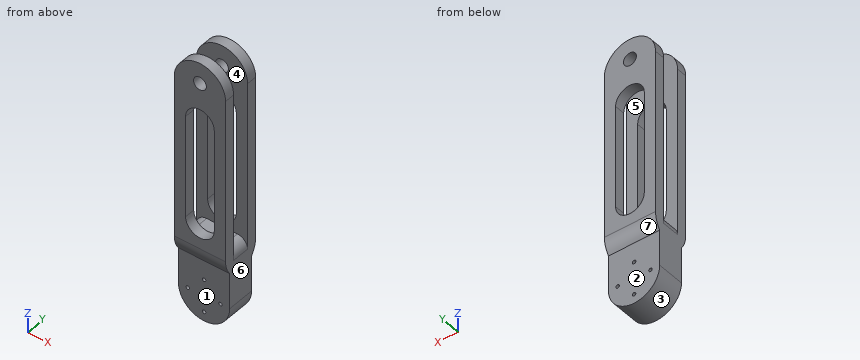
```python
from build123d import *

# Parameters (mm, degrees)
BOSS_EXTRU_1_DEPTH      = 12.5
CONG_1_R                = 12.5
ESQUISSE2_R             = 0.85
ENL_V_MAT_EXTRU_1_DEPTH = 122.715469949
ESQUISSE3_R             = 3.15
ENL_V_MAT_EXTRU_2_DEPTH = 123.082236628
ENL_V_MAT_EXTRU_3_DEPTH = 123.082236628
CONG_2_R                = 5


with BuildPart() as part:
    # Esquisse1 → Boss.-Extru.1 (new, symmetric)
    with BuildSketch(Plane(origin=(0, 0, 0), x_dir=(0, 0, -1), z_dir=(1, 0, 0))):
        Polygon((90, 9.325), (-10, 9.325), (-10, 4.325), (80, 4.325), (80, -4.325), (-10, -4.325), (-10, -9.325), (90, -9.325), (90, -6.75), (120, -6.75), (120, 6.75), (90, 6.75), align=None)
    extrude(amount=BOSS_EXTRU_1_DEPTH, both=True)

    # Congé1
    # the kernel refuses this fillet: 12.5 mm, written as the material it takes off along each edge
    with BuildSketch(Plane(origin=(-31.497429925, -9.325, -90), x_dir=(0, 1, 0), z_dir=(1, 0, 0))) as cong_1_piece_1:
        with BuildLine():
            CenterArc((12.5, 7.59897197), CONG_1_R, 180, 37.439095089)
            Line((0, 7.59897197), (-0.25, 7.59897197))
            Line((-0.25, 7.59897197), (-0.25, 0))
            Line((-0.25, 0), (0, -0.25))
            ThreePointArc((0, -0.25), (1.2875, -0.25), (2.3765, -0.151979439))
            Line((2.3765, -0.151979439), (2.575, 0))
        make_face()
    extrude(amount=62.99485985, mode=Mode.SUBTRACT)
    with BuildSketch(Plane(origin=(31.497429925, 9.325, -90), x_dir=(0, 0, 1), z_dir=(-1, 0, 0))) as cong_1_piece_2:
        with BuildLine():
            CenterArc((7.59897197, -12.5), CONG_1_R, 90, 37.439095089)
            Line((0, -2.575), (-0.151979439, -2.3765))
            ThreePointArc((-0.151979439, -2.3765), (-0.25, -1.2875), (-0.25, 0))
            Line((-0.25, 0), (0, 0.25))
            Line((0, 0.25), (7.59897197, 0.25))
            Line((7.59897197, 0.25), (7.59897197, 0))
        make_face()
    extrude(amount=62.99485985, mode=Mode.SUBTRACT)
    with BuildSketch(Plane(origin=(-12.5, 26.925, 10), x_dir=(1, 0, 0), z_dir=(0, -1, 0)), Plane(origin=(-12.5, 40.575, 10), x_dir=(1, 0, 0), z_dir=(0, -1, 0)), Plane(origin=(12.5, 40.575, 10), x_dir=(0, 0, -1), z_dir=(0, -1, 0))) as cong_1_piece_3:
        with BuildLine():
            CenterArc((CONG_1_R, -CONG_1_R), CONG_1_R, 90, 90)
            Line((0, -CONG_1_R), (-CONG_1_R * 0.02, -CONG_1_R))
            Line((-CONG_1_R * 0.02, -CONG_1_R), (-CONG_1_R * 0.02, CONG_1_R * 0.02))
            Line((-CONG_1_R * 0.02, CONG_1_R * 0.02), (CONG_1_R, CONG_1_R * 0.02))
            Line((CONG_1_R, CONG_1_R * 0.02), (CONG_1_R, 0))
        make_face()
    extrude(amount=67.5, mode=Mode.SUBTRACT)
    with BuildSketch(Plane(origin=(12.5, 26.925, 10), x_dir=(-1, 0, 0), z_dir=(0, -1, 0))) as cong_1_piece_4:
        with BuildLine():
            CenterArc((CONG_1_R, CONG_1_R), CONG_1_R, 180, 90)
            Line((0, CONG_1_R), (-CONG_1_R * 0.02, CONG_1_R))
            Line((-CONG_1_R * 0.02, CONG_1_R), (-CONG_1_R * 0.02, -CONG_1_R * 0.02))
            Line((-CONG_1_R * 0.02, -CONG_1_R * 0.02), (CONG_1_R, -CONG_1_R * 0.02))
            Line((CONG_1_R, -CONG_1_R * 0.02), (CONG_1_R, 0))
        make_face()
    extrude(amount=67.5, mode=Mode.SUBTRACT)
    with BuildSketch(Plane(origin=(-12.5, -38, -120), x_dir=(1, 0, 0), z_dir=(0, 1, 0))) as cong_1_piece_5:
        with BuildLine():
            CenterArc((CONG_1_R, -CONG_1_R), CONG_1_R, 90, 90)
            Line((0, -CONG_1_R), (-CONG_1_R * 0.02, -CONG_1_R))
            Line((-CONG_1_R * 0.02, -CONG_1_R), (-CONG_1_R * 0.02, CONG_1_R * 0.02))
            Line((-CONG_1_R * 0.02, CONG_1_R * 0.02), (CONG_1_R, CONG_1_R * 0.02))
            Line((CONG_1_R, CONG_1_R * 0.02), (CONG_1_R, 0))
        make_face()
    extrude(amount=76, mode=Mode.SUBTRACT)
    with BuildSketch(Plane(origin=(12.5, -38, -120), x_dir=(-1, 0, 0), z_dir=(0, 1, 0))) as cong_1_piece_6:
        with BuildLine():
            CenterArc((CONG_1_R, CONG_1_R), CONG_1_R, 180, 90)
            Line((0, CONG_1_R), (-CONG_1_R * 0.02, CONG_1_R))
            Line((-CONG_1_R * 0.02, CONG_1_R), (-CONG_1_R * 0.02, -CONG_1_R * 0.02))
            Line((-CONG_1_R * 0.02, -CONG_1_R * 0.02), (CONG_1_R, -CONG_1_R * 0.02))
            Line((CONG_1_R, -CONG_1_R * 0.02), (CONG_1_R, 0))
        make_face()
    extrude(amount=76, mode=Mode.SUBTRACT)

    # Esquisse2 → Enlèv. mat.-Extru.1 (cut, through all)
    with BuildSketch(Plane(origin=(0, 6.75, 0), x_dir=(1, 0, 0), z_dir=(0, 1, 0))):
        with Locations(Location((8, 107.5, 0), (0, 0, 270))):
            Circle(ESQUISSE2_R)
        with Locations(Location((0, 115.5, 0), (0, 0, 270))):
            Circle(ESQUISSE2_R)
        with Locations(Location((-8, 107.5, 0), (0, 0, 270))):
            Circle(ESQUISSE2_R)
        with Locations(Location((0, 99.5, 0), (0, 0, 270))):
            Circle(ESQUISSE2_R)
    extrude(amount=-ENL_V_MAT_EXTRU_1_DEPTH, mode=Mode.SUBTRACT)

    # Esquisse3 → Enlèv. mat.-Extru.2 (cut, through all)
    with BuildSketch(Plane(origin=(0, 9.325, 0), x_dir=(1, 0, 0), z_dir=(0, 1, 0))):
        with Locations(Location((0, 0, 0), (0, 0, 270))):
            Circle(ESQUISSE3_R)
    extrude(amount=-ENL_V_MAT_EXTRU_2_DEPTH, mode=Mode.SUBTRACT)

    # Esquisse4 → Enlèv. mat.-Extru.3 (cut, through all)
    with BuildSketch(Plane(origin=(0, 9.325, 0), x_dir=(1, 0, 0), z_dir=(0, 1, 0))):
        with BuildLine():
            Line((-7, 70), (-7, 20))
            ThreePointArc((-7, 20), (0, 13), (7, 20))
            Line((7, 20), (7, 70))
            ThreePointArc((7, 70), (0, 77), (-7, 70))
        make_face()
    extrude(amount=-ENL_V_MAT_EXTRU_3_DEPTH, mode=Mode.SUBTRACT)

    # Congé2
    cong_2_edges = [part.edges().sort_by_distance(p)[0] for p in [
        (12.5, 0, -80),
        (-12.5, 0, -80),
    ]]
    fillet(cong_2_edges, radius=CONG_2_R)


solid = part.part
```
The model under review builds one solid part; all positions refer to its coordinate system, in mm. Face numbers are marked on the shaded views. A direction names the side the tool comes from. Give positions to 0.01 mm unless a question says otherwise; leave off trailing zeros. Write each loop counter-clockwise with the first axis right and the second up, starting at its lowest first coordinate (ties: lowest second). Pieces come first, ordered by that corner, then holes. Notation, with made-up numbers: (66.5, -17) - (80.5, -17) arc R19 ccw to (80.5, 15) - close; hole circle Ø8 at (31.5, 31.5). An arc over 180 degrees is marked (long way). Answer in a Markdown table with one row per item. Add a question column.
1. Wall thickness on line 1 along X through (y, z) = (3.5, -107.5); line 2 along Y through (x, z) = (4.5, -9) (3 decimals); line 3 along X through (y, z) = (-7.5, -55): over which ranges is each line inside the solid? List them lowest first. Write a range as [from, to].
2. Draft analysis for pull direction Y (two halves, no side actions). For the marked faces 4, 5, 6 and 7, state which applies: +Y half, -Y half, draft (parallel to the pull), parting line (faces both ways), or undercut.
3. Tool access review of the marked faces 1, 2 and 3: name each direction out of +Z, -Z, +X, -X, +Y, -Y from which nothing blocks a thin tool from reaching the whole face with its end or side.
4. Insertion check: P1, Ø4, axis at x = 8, z = -93, coming from the +Y side; P2, Ø4.5, axis at x = 3.5, y = -1, coming from the +Z side; P3, Ø2, axis at x = -8, z = -107.5, coming from the -Y side. Each pin has a flat end and moves straight along its axis. Give the tip position at first contact, or say it passes through.
5. We need section D-D on z = 1. Write out the cut boundary in (x, y) (3 decimals), then the cut area to 3 significant figures.
6. We need section C-C on x = 4.5. Write out the cut boundary in (y, z) (3 decimals), then the cut area to 3 significant figures.
7. We need section A-A on z = -26.5. Write out the cut boundary in (x, y) (3 decimals).
8. We need section B-B on y = 5.5. Write out the cut boundary in (x, z).
Ans:
| question | item | result |
|---|---|---|
| 1 | line 1 | x = [-12.5, -8.85], [-7.15, 7.15], [8.85, 12.5] |
| 1 | line 2 | y = [-9.325, -4.325], [4.325, 9.325] |
| 1 | line 3 | x = [-12.5, -7], [7, 12.5] |
| 2 | face 4 | undercut |
| 2 | face 5 | undercut |
| 2 | face 6 | draft |
| 2 | face 7 | +Y half |
| 3 | face 1 | -Z, +X, -X, -Y |
| 3 | face 2 | -Z, +X, -X, +Y |
| 3 | face 3 | -Z, +Y, -Y |
| 4 | P1 | stops at y = 6.75 |
| 4 | P2 | stops at z = -80 |
| 4 | P3 | stops at y = -6.75 |
| 5 | outline | (-12, -9.325) - (-2.987, -9.325) - (-2.987, -4.325) - (-12, -4.325) - close; (-12, 4.325) - (-2.987, 4.325) - (-2.987, 9.325) - (-12, 9.325) - close; (2.987, -9.325) - (12, -9.325) - (12, -4.325) - (2.987, -4.325) - close; (2.987, 4.325) - (12, 4.325) - (12, 9.325) - (2.987, 9.325) - close |
| 5 | area | 180 mm^2 |
| 6 | outline | (-9.325, -82.401) arc R12.5 ccw to (-6.75, -90) - (-6.75, -119.162) - (6.75, -119.162) - (6.75, -90) arc R12.5 ccw to (9.325, -82.401) - (9.325, -75.362) - (4.325, -75.362) - (4.325, -80) - (-4.325, -80) - (-4.325, -75.362) - (-9.325, -75.362) - close; (-9.325, -14.638) - (-4.325, -14.638) - (-4.325, 9.162) - (-9.325, 9.162) - close; (4.325, -14.638) - (9.325, -14.638) - (9.325, 9.162) - (4.325, 9.162) - close |
| 6 | area | 852 mm^2 |
| 7 | outline | (-12.5, -9.325) - (-7, -9.325) - (-7, -4.325) - (-12.5, -4.325) - close; (-12.5, 4.325) - (-7, 4.325) - (-7, 9.325) - (-12.5, 9.325) - close; (7, -9.325) - (12.5, -9.325) - (12.5, -4.325) - (7, -4.325) - close; (7, 4.325) - (12.5, 4.325) - (12.5, 9.325) - (7, 9.325) - close |
| 8 | outline | (-12.5, -107.5) arc R12.5 ccw to (12.5, -107.5) - (12.5, -2.5) arc R12.5 ccw to (-12.5, -2.5) - close; hole circle Ø1.7 at (-8, -107.5); hole (-7, -70) arc R7 ccw to (7, -70) - (7, -20) arc R7 ccw to (-7, -20) - close; hole circle Ø6.3 at (0, 0); hole circle Ø1.7 at (0, -115.5); hole circle Ø1.7 at (0, -99.5); hole circle Ø1.7 at (8, -107.5) |
